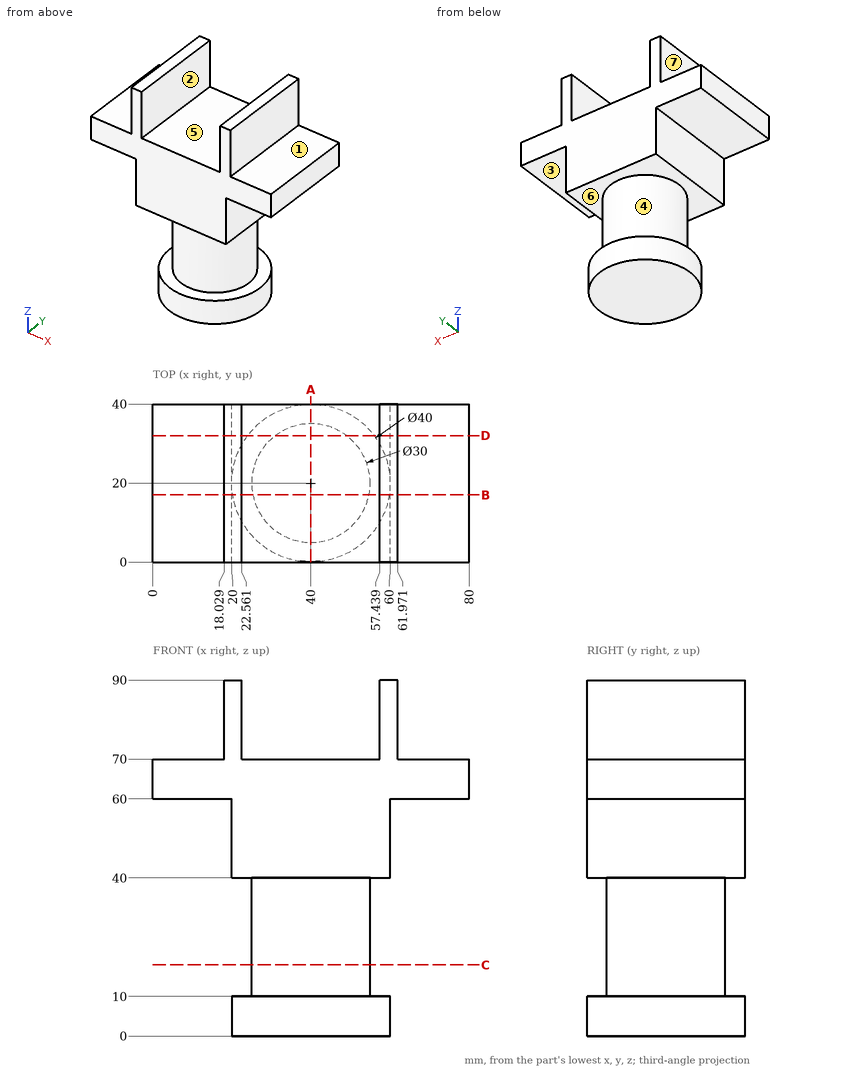
Drawing for the job (mm, zero at the part's lowest x, y, z). A direction names the side the tool comes from. Round coordinates to 2 decimals unless told otherwise and drop trailing zeros. Loops run counter-clockwise (first coordinate to the right, second up) from the corner with the lowest first, then second, coordinate; pieces in that order, holes last. Notation, with made-up numbers: (26, 31.25) -> (74, 31.25) arc R16 cw to (74, 55.25) -> close; hole circle Ø7 at (32, 76.25). An arc over 180 degrees is marked (long way). Use one line per item in the form item = value. Start each with the question number.
Item 1: Band-saw the part on B-B (y = 17). List the corners of the cut face in (x, z), plus the area to 3 significant figures.
Item 2: Tool access for the marked faces 1, 2, 3 and 4: list every direction of +Z, -Z, +X, -X, +Y, -Y with a clear straight run to the whole face (end or side of a thin tool).
Item 3: Band-saw the part on C-C (z = 18). List the corners of the cut face in (x, y), plus the area to 3 significant figures.
Item 4: Two-plate mould, pull along X, no slides. Class the marked faces 5, 6 and 7: released by +X, released by -X, zero draft, split by the parting line, or undercut.
Item 5: Band-saw the part on D-D (y = 32). List the corners of the cut face in (x, z), plus the area to 3 significant figures.
Item 6: Band-saw the part on A-A (x = 40). List the corners of the cut face in (y, z), plus the area to 3 significant figures.
Item 7: Drop flat-ended pins along their axis: pin 1 Ø4 at (x, z) = (26, 44.5) entering from -Y; pin 2 Ø1 at (x, z) = (48.5, 15.5) entering from +Y; pin 3 Ø22 at (y, z) = (28.5, 47) entering from -X; pin 4 Ø6 at (x, y) = (74, 24.5) entering from -Z. Give the stop position or say it passes through.
Item 8: Drill centre lines: line 1 along X through (y, z) = (15.5, 77); line 2 along Z through (x, y) = (54.5, 26); line 3 along Z through (x, y) = (64.5, 8.5). Where is each one in solid material? Low to high.
Data:
q1.outline = (0, 60) -> (20, 60) -> (20, 40) -> (25.3, 40) -> (25.3, 10) -> (20.23, 10) -> (20.23, 0) -> (59.77, 0) -> (59.77, 10) -> (54.7, 10) -> (54.7, 40) -> (60, 40) -> (60, 60) -> (80, 60) -> (80, 70) -> (61.97, 70) -> (61.97, 90) -> (57.44, 90) -> (57.44, 70) -> (22.56, 70) -> (22.56, 90) -> (18.03, 90) -> (18.03, 70) -> (0, 70) -> close
q1.area = 3,060 mm^2
q2.face_1 = +Z, +X, +Y, -Y
q2.face_2 = +Z, +Y, -Y
q2.face_3 = -Z, +X, +Y, -Y
q2.face_4 = none
q3.outline = circle Ø30 at (40, 20)
q3.area = 707 mm^2
q4.face_5 = undercut
q4.face_6 = zero draft
q4.face_7 = released by -X
q5.outline = (0, 60) -> (20, 60) -> (20, 40) -> (31, 40) -> (31, 10) -> (24, 10) -> (24, 0) -> (56, 0) -> (56, 10) -> (49, 10) -> (49, 40) -> (60, 40) -> (60, 60) -> (80, 60) -> (80, 70) -> (61.97, 70) -> (61.97, 90) -> (57.44, 90) -> (57.44, 70) -> (22.56, 70) -> (22.56, 90) -> (18.03, 90) -> (18.03, 70) -> (0, 70) -> close
q5.area = 2,640 mm^2
q6.outline = (0, 0) -> (40, 0) -> (40, 10) -> (35, 10) -> (35, 40) -> (40, 40) -> (40, 70) -> (0, 70) -> (0, 40) -> (5, 40) -> (5, 10) -> (0, 10) -> close
q6.area = 2,500 mm^2
q7.pin_1 = 0
q7.pin_2 = 32.69
q7.pin_3 = 20
q7.pin_4 = 60
q8.line_1 = 18.03 to 22.56, 57.44 to 61.97
q8.line_2 = 0 to 10, 40 to 70
q8.line_3 = 60 to 70
